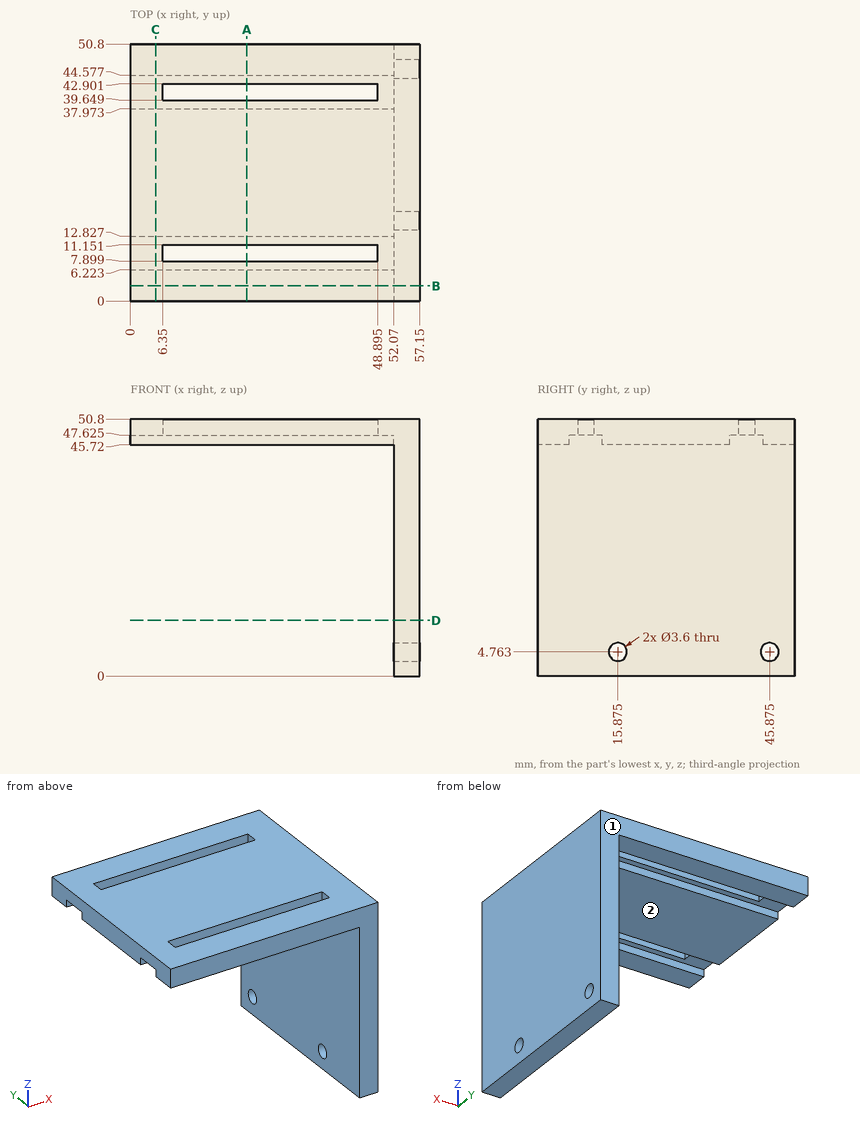
The drawing under review shows one solid part. Ordinate dimensions are in mm from its lowest x, y, z. A direction names the side the tool comes from. Coordinates: 2 decimals unless noted, no trailing zeros. Write each loop counter-clockwise with the first axis right and the second up, starting at its lowest first coordinate (ties: lowest second). Pieces come first, ordered by that corner, then holes. Notation, with made-up numbers: (-20, 17) - (36, 17) arc R26 ccw to (36, 39) - close; hole circle Ø1 at (77.5, 89.25). An arc over 180 degrees is marked (long way). Answer in a Markdown table with one row per item. Add a question column.
Q1. For P1, Ø20, axis at x = 29, y = 29, coming from the -Z side; P2, Ø2, axis at x = 25.5, y = 39.5, coming from the -Z side (1 decimal); P3, Ø4, axis at y = 45.88, z = 4.76, coming from the -X side, all flat-tipped, find the tip position at first contact; note any pin that passes through.
Q2. We need section D-D, the plane z = 11. State the section outline as (x, y) points, and give its area (3 significant figures).
Q3. We need section B-B, the plane y = 3. State the section outline as (x, z) points.
Q4. For probe 1 along X at (y, z) = (4, 45); probe 2 along Z at (x, y) = (31.5, 7) (1 decimal); probe 3 along Z at (x, y) = (27.5, 35), list the stretches that pass through material, from the lowest coordinate up.
Q5. We need section A-A, the plane x = 23. Count the separate pieces of the cut face and the enclosed holes in it, and give its area (3 significant figures).
Q6. Tool access review of the marked faces 1 and 2: name each direction out of +Z, -Z, +X, -X, +Y, -Y from which nothing blocks a thin tool from reaching the whole face with its end or side.
Q7. We need section C-C, the plane x = 5. State the section outline as (y, z) points (1 decimal).
Answer list:
| question | item | result |
|---|---|---|
| 1 | P1 | stops at z = 45.72 |
| 1 | P2 | stops at z = 47.6 |
| 1 | P3 | stops at x = 52.07 |
| 2 | outline | (52.07, 0) - (57.15, 0) - (57.15, 50.8) - (52.07, 50.8) - close |
| 2 | area | 258 mm2 |
| 3 | outline | (0, 45.72) - (52.07, 45.72) - (52.07, 0) - (57.15, 0) - (57.15, 50.8) - (0, 50.8) - close |
| 4 | probe 1 | x = 52.07 to 57.15 |
| 4 | probe 2 | z = 47.6 to 50.8 |
| 4 | probe 3 | z = 45.72 to 50.8 |
| 5 | separate pieces | 3 |
| 5 | enclosed holes | 0 |
| 5 | area | 212 mm2 |
| 6 | face 1 | +Z, -Z, +X, -X, +Y |
| 6 | face 2 | -Z, -X, +Y, -Y |
| 7 | outline | (0, 45.7) - (6.2, 45.7) - (6.2, 47.6) - (12.8, 47.6) - (12.8, 45.7) - (38, 45.7) - (38, 47.6) - (44.6, 47.6) - (44.6, 45.7) - (50.8, 45.7) - (50.8, 50.8) - (0, 50.8) - close |
